from build123d import *

# Parameters (mm, degrees)
REPISA_M4_START                       = 222.25
REPISA_M4_DEPTH                       = 6.35
BARRENOS_M4_TORNILLOS_PASADORES_START = 222.25
CROQUIS2_R                            = 1.45
CROQUIS2_R_2                          = 8
CROQUIS2_R_3                          = 1.7
CROQUIS2_R_4                          = 1.5
BARRENOS_M4_TORNILLOS_PASADORES_DEPTH = 6.35
REFRENTADO_M2_5_START                 = 222.25
CROQUIS3_R                            = 2.5
REFRENTADO_M2_5_DEPTH                 = 2.6
AVELLANADO_M3_START                   = 226.9
CROQUIS4_R                            = 3.15
AVELLANADO_M3_DEPTH                   = 1.7


with BuildPart() as part:
    # Croquis1 → Repisa_M4 (new body)
    with BuildSketch(Plane.XY.offset(REPISA_M4_START)):
        with BuildLine():
            Line((126.4, -30), (178.4, -30))
            ThreePointArc((178.4, -30), (182.642640687, -28.242640687), (184.4, -24))
            Line((184.4, -24), (184.4, 24))
            ThreePointArc((184.4, 24), (182.642640687, 28.242640687), (178.4, 30))
            Line((178.4, 30), (126.4, 30))
            ThreePointArc((126.4, 30), (122.157359313, 28.242640687), (120.4, 24))
            Line((120.4, 24), (120.4, -24))
            ThreePointArc((120.4, -24), (122.157359313, -28.242640687), (126.4, -30))
        make_face()
    extrude(amount=REPISA_M4_DEPTH)

    # Croquis2 → Barrenos_M4_tornillos_pasadores (cut)
    with BuildSketch(Plane.XY.offset(BARRENOS_M4_TORNILLOS_PASADORES_START)):
        with Locations((172.863916472, 1.215780658)):
            Circle(CROQUIS2_R)
        with Locations((161.579061301, 18.330161855)):
            Circle(CROQUIS2_R)
        with Locations((141.115144828, 17.114381197)):
            Circle(CROQUIS2_R)
        with Locations((131.936083528, -1.215780658)):
            Circle(CROQUIS2_R)
        with Locations((143.220938699, -18.330161855)):
            Circle(CROQUIS2_R)
        with Locations((163.684855172, -17.114381197)):
            Circle(CROQUIS2_R)
        with Locations((152.4, 0)):
            Circle(CROQUIS2_R_2)
        with Locations((125.4, 0)):
            Circle(CROQUIS2_R_3)
        with Locations((179.4, 0)):
            Circle(CROQUIS2_R_3)
        with Locations((138.4, 0)):
            Circle(CROQUIS2_R_4)
        with Locations((166.4, 0)):
            Circle(CROQUIS2_R_4)
    extrude(amount=BARRENOS_M4_TORNILLOS_PASADORES_DEPTH, mode=Mode.SUBTRACT)

    # Croquis3 → Refrentado_M2-5 (cut)
    with BuildSketch(Plane.XY.offset(REFRENTADO_M2_5_START)):
        with Locations((172.863916472, 1.215780658)):
            Circle(CROQUIS3_R)
        with Locations((161.579061301, 18.330161855)):
            Circle(CROQUIS3_R)
        with Locations((141.115144828, 17.114381197)):
            Circle(CROQUIS3_R)
        with Locations((131.936083528, -1.215780658)):
            Circle(CROQUIS3_R)
        with Locations((143.220938699, -18.330161855)):
            Circle(CROQUIS3_R)
        with Locations((163.684855172, -17.114381197)):
            Circle(CROQUIS3_R)
    extrude(amount=REFRENTADO_M2_5_DEPTH, mode=Mode.SUBTRACT)

    # Croquis4 → Avellanado_M3 (cut)
    with BuildSketch(Plane.XY.offset(AVELLANADO_M3_START)):
        with Locations(Location((125.4, 0, 0), (0, 0, 180))):
            Circle(CROQUIS4_R)
        with Locations(Location((179.4, 0, 0), (0, 0, 180))):
            Circle(CROQUIS4_R)
    extrude(amount=AVELLANADO_M3_DEPTH, mode=Mode.SUBTRACT)


solid = part.part
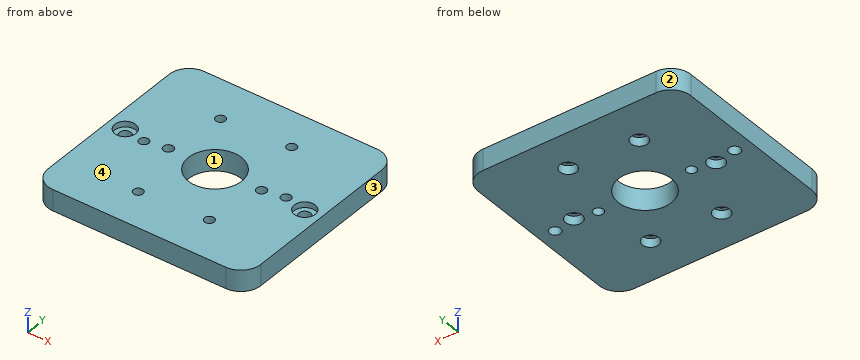
Build history of the part. All positions in model axes, mm. Face numbers are marked on the shaded views. Round coordinates to 2 decimals unless told otherwise and drop trailing zeros. Write each loop counter-clockwise with the first axis right and the second up, starting at its lowest first coordinate (ties: lowest second). Pieces come first, ordered by that corner, then holes. Notation, with made-up numbers: (1, -14) - (22, -14) arc R4 cw to (22, -7) - close; hole circle Ø1 at (0.25, 86). An arc over 180 degrees is marked (long way). Use CSV: the item, a comma, the result in double quotes.
(1) Band-saw the part on A-A (x = 152.4). Write the cut outline in (y, z).
Response:
outline,"(-30, 222.25) - (-8, 222.25) - (-8, 228.6) - (-30, 228.6) - close; (8, 222.25) - (30, 222.25) - (30, 228.6) - (8, 228.6) - close"
(2) Pin check, flat tip, straight feed: P1, Ø2.5, axis at x = 142, y = 17, coming from the -Z side. Stop position of the tip, or through.
Response:
P1,"z = 224.85"
(3) Wall check: line 1 (Y direction, x = 173, z = 223.75); line 2 (Y direction, x = 166.5, z = 225.75); line 3 (X direction, y = -19.5, z = 227.5). Give the ranges that are in metal, low to high.
Response:
line 1,"-30 to -1.28, 3.71 to 30"
line 2,"-30 to -1.5, 1.5 to 30"
line 3,"120.4 to 142.36, 144.08 to 184.4"
(4) Band-saw the part on B-B (z = 223). Give the number of separate pieces and of enclosed holes in the cut face, plus the area to 3 significant figures.
Response:
separate pieces,"1"
enclosed holes,"11"
area,"3,460 mm²"
(5) Band-saw the part on D-D (x = 179.4). Write the cut outline in (y, z).
Response:
outline,"(-29.92, 222.25) - (-1.7, 222.25) - (-1.7, 226.9) - (-3.15, 226.9) - (-3.15, 228.6) - (-29.92, 228.6) - close; (1.7, 222.25) - (29.92, 222.25) - (29.92, 228.6) - (3.15, 228.6) - (3.15, 226.9) - (1.7, 226.9) - close"
(6) Band-saw the part on C-C (x = 172.5). Write the cut outline in (y, z), plus the area to 3 significant figures.
Response:
outline,"(-30, 222.25) - (-1.26, 222.25) - (-1.26, 224.85) - (-0.19, 224.85) - (-0.19, 228.6) - (-30, 228.6) - close; (2.62, 224.85) - (3.69, 224.85) - (3.69, 222.25) - (30, 222.25) - (30, 228.6) - (2.62, 228.6) - close"
area,"358 mm²"
(7) Mould opens along X. For the marked faces 1, 2, 3 and 4 say: pulls with the +X half, pulls with the -X half, needs draft (parallel to the pull), parting line crosses it, or undercut.
Response:
face 1,"undercut"
face 2,"pulls with the -X half"
face 3,"pulls with the +X half"
face 4,"needs draft"
